Can you work these out from the drawing? Everything is in mm from the part's minimum corner. Give positions to 0.01 mm unless a question says otherwise; leave off trailing zeros. Loops run counter-clockwise (first coordinate to the right, second up) from the corner with the lowest first, then second, coordinate; pieces in that order, holes last. Notation, with made-up numbers: (-16, 24) -> (30, 24) arc R33 ccw to (30, 58) -> close; hole circle Ø8 at (58.5, 12.5). An arc over 180 degrees is marked (long way). Return JSON: item names as keys, results as strings. Group by question number.
Q1. Will these pins go through, and if not, where does the flat tip stop? pin 1 (8 mm diameter, centred on x = 40, z = 17, fed in from -Y); pin 2 (3 mm diameter, centred on y = 159, z = 15.5, fed in from -X) (1 decimal); pin 3 (3 mm diameter, centred on x = 119, y = 23.5, fed in from -Z) (1 decimal).
Q2. Suppose I cut it at B-B, the plane z = 27. Please give me the cut outline in (x, y).
Q3. I need wall thicknesses on line 1 along X through (y, z) = (67, 8) (1 decimal); line 2 along X through (y, z) = (25, 12) (1 decimal); line 3 along Z through (x, y) = (89, 178.5) (1 decimal). Which ranges of each line are inside material? Lowest first, please. Write a range as [from, to].
Q4. Suppose I cut it at A-A, the plane y = 119. Please give me the cut outline in (x, z) (1 decimal), and give its area (3 significant figures).
Q5. Suppose I cut it at C-C, the plane x = 16. Please give me the cut outline in (y, z), and give its area (3 significant figures).
Q6. Thinking about a two-plate mould opening in X: for the marked faces 1, 2 and 3, which applies, pulls with the +X half, pulls with the -X half, needs draft (parallel to the pull), parting line crosses it, or undercut?
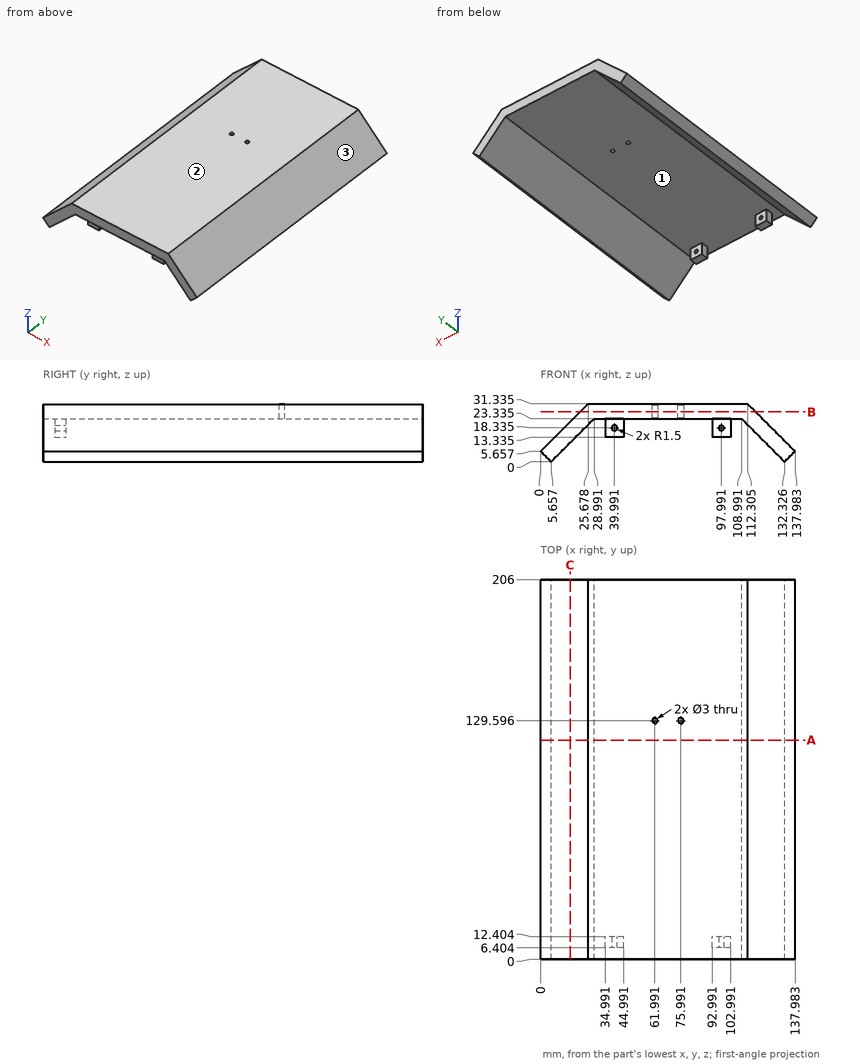
Ans:
{
 "1": {"pin 1": "stops at y = 6.4", "pin 2": "stops at x = 8.3", "pin 3": "stops at z = 11.8"},
 "2": {"outline": "(21.34, 0) -> (116.64, 0) -> (116.64, 206) -> (21.34, 206) -> close; hole circle Ø3 at (61.99, 129.6); hole circle Ø3 at (75.99, 129.6)"},
 "3": {"line 1": "x = [2.3, 13.7], [124.3, 135.6]", "line 2": "x = [6.3, 17.7], [120.3, 131.6]", "line 3": "z = [23.3, 31.3]"},
 "4": {"outline": "(0, 5.7) -> (5.7, 0) -> (29, 23.3) -> (109, 23.3) -> (132.3, 0) -> (138, 5.7) -> (112.3, 31.3) -> (25.7, 31.3) -> close", "area": "1,220 mm^2"},
 "5": {"outline": "(0, 10.34) -> (206, 10.34) -> (206, 21.66) -> (0, 21.66) -> close", "area": "2,330 mm^2"},
 "6": {"face 1": "undercut", "face 2": "needs draft", "face 3": "pulls with the +X half"}
}
